Build history of the part. All positions in model axes, mm. Face numbers are marked on the shaded views. A direction names the side the tool comes from. Give positions to 0.01 mm unless a question says otherwise; leave off trailing zeros. Loops run counter-clockwise (first coordinate to the right, second up) from the corner with the lowest first, then second, coordinate; pieces in that order, holes last. Notation, with made-up numbers: M 13.25,-35 L 27.25,-35 A16 ccw 27.25,-13 Z; hole C 24.5,84 d9. An arc over 180 degrees is marked long. Answer as a JSON object with one key per item and string values. Group by question number.
1. Slice it at A-A (z = 116.6). List the corners of the cut face in (x, y), then the cut area to 3 significant figures.
2. Drill centre lines: line 1 along Y through (x, z) = (-39.25, 129.1); line 2 along X through (y, z) = (-38, 129.1); line 3 along X through (y, z) = (4.5, 98). Where is each one in solid material? Low to high. Write a range as [from, to].
3. Drop flat-ended pins along their axis: pin 1 Ø7 at (x, z) = (21, 64.5) entering from -Y; pin 2 Ø2.5 at (y, z) = (-29, 64.5) entering from +X. Give the stop position or say it passes through.
4. Slice it at D-D (y = -11). List the corners of the cut face in (x, z), then the cut area to 3 significant figures.
5. Slice it at B-B (y = -29). List the corners of the cut face in (x, z), then the cut area to 3 significant figures.
6. 3-axis set-ups, long thin cutter, end or side, ignore diameter. For the marked faces 4 and 5: which of +Z, -Z, +X, -X, +Y, -Y reach the whole face in a straight line?
7. Mould opens along X. For the marked faces 1, 2 and 3 say: released by +X, released by -X, zero draft, split by the parting line, or undercut.
from build123d import *

# Parameters (mm, degrees)
SKETCH1_W                      = 80
SKETCH1_H                      = 80
SKETCH1_W_2                    = 74
SKETCH1_H_2                    = 74
BOSS_EXTRUDE1_DEPTH            = 79.6
M4_CLEARANCE_HOLE1_D           = 4.5
M4_CLEARANCE_HOLE1_ON_FACE_2_D = 4.5
M4_CLEARANCE_HOLE1_ON_FACE_3_D = 4.5
M4_CLEARANCE_HOLE1_ON_FACE_4_D = 4.5
F_3_0_3_DIAMETER_HOLE1_D       = 3
F_3_0_3_DIAMETER_HOLE1_DEPTH   = 3


with BuildPart() as part:
    # Sketch1 → Boss-Extrude1 (new body)
    with BuildSketch(Plane.XY.offset(57)):
        Rectangle(SKETCH1_W, SKETCH1_H)
        Rectangle(SKETCH1_W_2, SKETCH1_H_2, mode=Mode.SUBTRACT)
    extrude(amount=BOSS_EXTRUDE1_DEPTH)

    # M4 Clearance Hole1 (through all)
    with Locations(Plane(origin=(40, 29, 64.5), x_dir=(0, 0, 1), z_dir=(1, 0, 0))):
        with Locations((0, 0), (0, 58), (0, 29), (64.6, 0), (64.6, 29), (64.6, 58)):
            Hole(M4_CLEARANCE_HOLE1_D / 2)

    # M4 Clearance Hole1 on face 2 (through all)
    with Locations(Plane(origin=(21, 40, 64.5), x_dir=(0, 0, 1), z_dir=(0, 1, 0))):
        with Locations((0, 0), (0, -42), (64.6, -42), (64.6, 0)):
            Hole(M4_CLEARANCE_HOLE1_ON_FACE_2_D / 2)

    # M4 Clearance Hole1 on face 3 (through all)
    with Locations(Plane(origin=(-40, 29, 64.5), x_dir=(0, 0, -1), z_dir=(-1, 0, 0))):
        with Locations((0, 0), (0, 29), (0, 58), (-64.6, 58), (-64.6, 29), (-64.6, 0)):
            Hole(M4_CLEARANCE_HOLE1_ON_FACE_3_D / 2)

    # M4 Clearance Hole1 on face 4 (through all)
    with Locations(Plane(origin=(21, -40, 64.5), x_dir=(0, 0, -1), z_dir=(0, -1, 0))):
        with Locations((0, 0), (0, -42), (-64.6, -42), (-64.6, 0)):
            Hole(M4_CLEARANCE_HOLE1_ON_FACE_4_D / 2)

    # Ø3.0 (3) Diameter Hole1
    with Locations(Plane(origin=(40, 0, 0), x_dir=(0, 0, -1), z_dir=(1, 0, 0))):
        with Locations((-77, 30), (-116.6, 24), (-116.6, 30), (-77, 24)):
            Hole(F_3_0_3_DIAMETER_HOLE1_D / 2, depth=F_3_0_3_DIAMETER_HOLE1_DEPTH)


solid = part.part
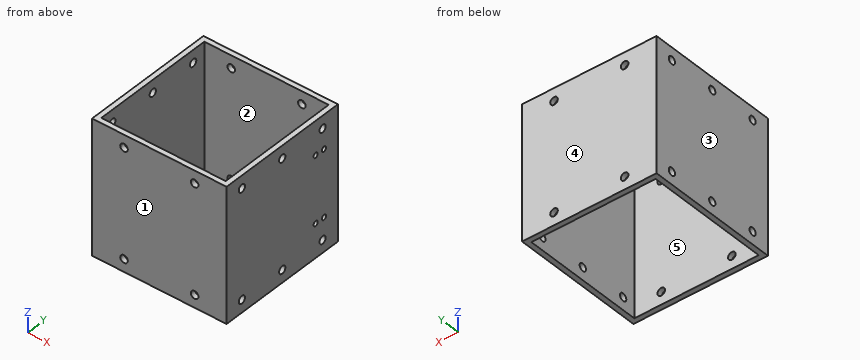
Established:
{
 "1": {"outline": "M -40,-40 L 40,-40 L 40,22.5 L 37,22.5 L 37,-37 L -37,-37 L -37,37 L 37,37 L 37,31.5 L 40,31.5 L 40,40 L -40,40 Z; M 37,25.5 L 40,25.5 L 40,28.5 L 37,28.5 Z", "area": "906 mm^2"},
 "2": {"line 1": "y = [-40, -31.25], [-26.75, -2.25], [2.25, 26.75], [31.25, 40]", "line 2": "x = [-40, -23.25], [-18.75, 18.75], [23.25, 40]", "line 3": "x = [-40, -37], [37, 40]"},
 "3": {"pin 1": "stops at y = -40", "pin 2": "passes through"},
 "4": {"outline": "M -40,57 L -37,57 L -37,136.6 L -40,136.6 Z; M 37,57 L 40,57 L 40,136.6 L 37,136.6 Z", "area": "478 mm^2"},
 "5": {"outline": "M -40,57 L -37,57 L -37,62.25 L -40,62.25 Z; M -40,66.75 L -37,66.75 L -37,126.85 L -40,126.85 Z; M -40,131.35 L -37,131.35 L -37,136.6 L -40,136.6 Z; M 37,57 L 40,57 L 40,62.25 L 37,62.25 Z; M 37,66.75 L 40,66.75 L 40,126.85 L 37,126.85 Z; M 37,131.35 L 40,131.35 L 40,136.6 L 37,136.6 Z", "area": "424 mm^2"},
 "6": {"face 4": "+Z, -Z, +X, -X, +Y", "face 5": "+Z, -Z"},
 "7": {"face 1": "zero draft", "face 2": "undercut", "face 3": "released by -X"}
}
